For this review, take the finished solid that the model builds, in its own axes (mm). Face numbers are marked on the shaded views. A direction names the side the tool comes from. Round coordinates to 2 decimals unless told otherwise and drop trailing zeros. Loops run counter-clockwise (first coordinate to the right, second up) from the corner with the lowest first, then second, coordinate; pieces in that order, holes last.
1. To check wall thickness, follow line 1 along Y through (x, z) = (-16.75, -2.5); line 2 along Z through (x, y) = (-20.5, 4.5); line 3 along Z through (x, y) = (-17.75, 2). State the ranges of each line that lie inside material, in increasing order.
2. Tool access review of the marked faces 1, 2 and 3: name each direction out of +Z, -Z, +X, -X, +Y, -Y from which nothing blocks a thin tool from reaching the whole face with its end or side.
3. Consider section C-C on z = -0.25. State the section outline as (x, y) points, then the cut area to 3 significant figures.
4. Consider section A-A on z = 3.75. State the section outline as (x, y) points.
5. Clearance check with flat-ended pins moving along their axes: pin 1 Ø5 at (x, z) = (-12.71, 3.15) entering from -Y; pin 2 Ø2.5 at (x, z) = (-12.71, -10.36) entering from +Y; pin 3 Ø2 at (y, z) = (7, -0.5) entering from +X; pin 4 Ø6 at (x, z) = (-14.5, -9.5) entering from +Y. State where each tip first meets the part, or that it passes through.
6. Consider section B-B on x = -33.25. State the section outline as (y, z) points.
7. Consider section D-D on y = 7.5. State the section outline as (x, z) points (3 decimals).
from build123d import *

# Parameters (mm, degrees)
BOSS_EXTRUDE1_DEPTH = 1
SKETCH2_R           = 9.305
BOSS_EXTRUDE2_DEPTH = 13.66
SKETCH3_R           = 3.1
BOSS_EXTRUDE3_DEPTH = 8.51
SKETCH4_R           = 1.485
CUT_EXTRUDE1_DEPTH  = 8.51


with BuildPart() as part:
    # Sketch1 → Boss-Extrude1 (new body)
    with BuildSketch(Plane(origin=(0, 0, 0), x_dir=(1, 0, 0), z_dir=(0, 1, 0))):
        with BuildLine():
            Line((-13.933041308, 13.509742501), (-28.57709975, 13.509742501))
            ThreePointArc((-28.57709975, 13.509742501), (-38.47709975, 3.609742501), (-28.57709975, -6.290257499))
            Line((-28.57709975, -6.290257499), (-13.933041308, -6.290257499))
            ThreePointArc((-13.933041308, -6.290257499), (-10.908622294, -4.147777693), (-11.926545628, -0.583908702))
            Line((-11.926545628, -0.583908702), (-14.03709975, 1.109742501))
            Line((-14.03709975, 1.109742501), (-14.03709975, 6.109742501))
            Line((-14.03709975, 6.109742501), (-11.926545628, 7.803393704))
            ThreePointArc((-11.926545628, 7.803393704), (-10.908622294, 11.367262695), (-13.933041308, 13.509742501))
        make_face()
    extrude(amount=BOSS_EXTRUDE1_DEPTH)

    # Sketch2 → Boss-Extrude2 (add)
    with BuildSketch(Plane(origin=(0, 1, 0), x_dir=(1, 0, 0), z_dir=(0, 1, 0))):
        with Locations(Location((-28.57709975, 3.609742501, 0), (0, 0, 270))):
            Circle(SKETCH2_R)
    extrude(amount=BOSS_EXTRUDE2_DEPTH)

    # Sketch3 → Boss-Extrude3 (add)
    with BuildSketch(Plane(origin=(0, 1, 0), x_dir=(1, 0, 0), z_dir=(0, 1, 0))):
        with Locations(Location((-17.962659231, 10.215706191, 0), (0, 0, 270))):
            Circle(SKETCH3_R)
    extrude(amount=BOSS_EXTRUDE3_DEPTH)

    # Sketch4 → Cut-Extrude1 (cut)
    with BuildSketch(Plane(origin=(0, 1, 0), x_dir=(1, 0, 0), z_dir=(0, 1, 0))):
        with Locations(Location((-12.71209975, 10.364742501, 0), (0, 0, 270))):
            Circle(SKETCH4_R)
        with Locations(Location((-12.71209975, -3.145257499, 0), (0, 0, 270))):
            Circle(SKETCH4_R)
    extrude(amount=-CUT_EXTRUDE1_DEPTH, mode=Mode.SUBTRACT)


solid = part.part
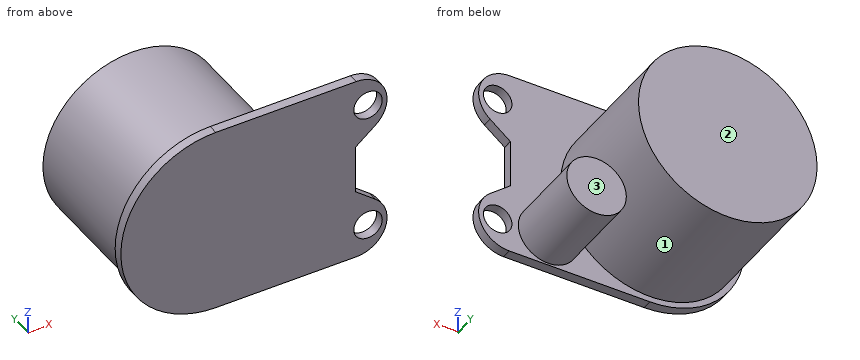
Resolved:
1. line 1: y = 0 to 1
1. line 2: z = -12 to -8.43, -8.23 to 1.01
1. line 3: z = -13.31 to -7.12
2. face 1: +Y
2. face 2: +Z, -Z, +X, -X, +Y
2. face 3: -Z, +X, +Y
3. outline: (-37.89, 0) - (-12.97, 0) - (-12.97, 1) - (-19.9, 1) - (-19.9, 14.66) - (-37.25, 14.66) - (-37.25, 1) - (-37.89, 1) - close
3. area: 262 mm2
4. outline: (-35.2, 0) - (-14.07, 0) - (-14.07, 1) - (-22.88, 1) - (-22.88, 14.66) - (-34.27, 14.66) - (-34.27, 1) - (-35.2, 1) - close; (-11.36, 0) - (-10.8, 0) - (-10.8, 1) - (-11.36, 1) - close
5. pin 1: stops at y = 0
5. pin 2: passes through
5. pin 3: stops at x = -19.51
5. pin 4: stops at y = 9.51
6. outline: (0, -12.34) - (1, -12.34) - (1, -11.66) - (14.66, -11.66) - (14.66, 4.44) - (1, 4.44) - (1, 5.12) - (0, 5.12) - close
7. outline: circle Ø18.61 at (-28.577, -3.61); circle Ø6.2 at (-17.963, -10.216)
